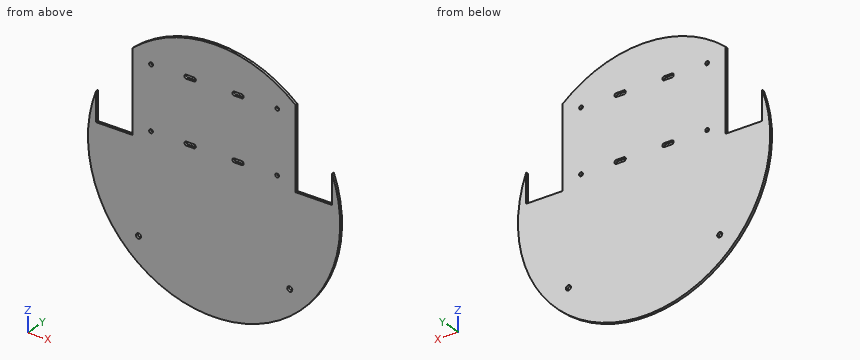
```python
from build123d import *

# Parameters (mm, degrees)
SKETCH1_R           = 1.5
SKETCH1_R_2         = 2
BOSS_EXTRUDE1_DEPTH = 2


with BuildPart() as part:
    # Sketch1 → Boss-Extrude1 (new body)
    with BuildSketch(Plane(origin=(0, 0, 0), x_dir=(1, 0, 0), z_dir=(0, 1, 0))):
        with BuildLine():
            Line((-93.5, -35.464771253), (-93.5, -12.5))
            Line((-93.5, -12.5), (-64.5, -12.5))
            Line((-64.5, -12.5), (-64.5, -76.418256981))
            ThreePointArc((-64.5, -76.418256981), (0, -100), (64.5, -76.418256981))
            Line((64.5, -76.418256981), (64.5, -12.5))
            Line((64.5, -12.5), (93.5, -12.5))
            Line((93.5, -12.5), (93.5, -35.464771253))
            ThreePointArc((93.5, -35.464771253), (0, 100), (-93.5, -35.464771253))
        make_face()
        with Locations((-50, -69)):
            Circle(SKETCH1_R, mode=Mode.SUBTRACT)
        with BuildLine():
            Line((-22, -67.5), (-16, -67.5))
            ThreePointArc((-16, -67.5), (-14.5, -69), (-16, -70.5))
            Line((-16, -70.5), (-22, -70.5))
            ThreePointArc((-22, -70.5), (-23.5, -69), (-22, -67.5))
        make_face(mode=Mode.SUBTRACT)
        with Locations((-50, -20)):
            Circle(SKETCH1_R, mode=Mode.SUBTRACT)
        with BuildLine():
            ThreePointArc((-16, -18.5), (-14.5, -20), (-16, -21.5))
            Line((-16, -21.5), (-22, -21.5))
            ThreePointArc((-22, -21.5), (-23.5, -20), (-22, -18.5))
            Line((-22, -18.5), (-16, -18.5))
        make_face(mode=Mode.SUBTRACT)
        with BuildLine():
            ThreePointArc((16, -70.5), (14.5, -69), (16, -67.5))
            Line((16, -67.5), (22, -67.5))
            ThreePointArc((22, -67.5), (23.5, -69), (22, -70.5))
            Line((22, -70.5), (16, -70.5))
        make_face(mode=Mode.SUBTRACT)
        with Locations((50, -69)):
            Circle(SKETCH1_R, mode=Mode.SUBTRACT)
        with BuildLine():
            Line((22, -21.5), (16, -21.5))
            ThreePointArc((16, -21.5), (14.5, -20), (16, -18.5))
            Line((16, -18.5), (22, -18.5))
            ThreePointArc((22, -18.5), (23.5, -20), (22, -21.5))
        make_face(mode=Mode.SUBTRACT)
        with Locations((50, -20)):
            Circle(SKETCH1_R, mode=Mode.SUBTRACT)
        with Locations((-60, 60)):
            Circle(SKETCH1_R_2, mode=Mode.SUBTRACT)
        with Locations((60, 60)):
            Circle(SKETCH1_R_2, mode=Mode.SUBTRACT)
    extrude(amount=BOSS_EXTRUDE1_DEPTH)


solid = part.part
```
Here's how the part is built. I have some questions about the finished solid (model axes, mm). Give positions to 0.01 mm unless a question says otherwise; leave off trailing zeros. Write each loop counter-clockwise with the first axis right and the second up, starting at its lowest first coordinate (ties: lowest second). Pieces come first, ordered by that corner, then holes. Notation, with made-up numbers: M -25,-28.5 L -8,-28.5 A18 cw -8,-0.5 Z; hole C 14,13.25 d11. An arc over 180 degrees is marked long. Put each result on its own line as item: value. Start each with the question number.
Item 1: Will these pins go through, and if not, where does the flat tip stop? pin 1 (2.5 mm diameter, centred on x = 50, z = 20, fed in from -Y); pin 2 (0.6 mm diameter, centred on x = 19, y = 0.5, fed in from -Z); pin 3 (0.6 mm diameter, centred on x = -20, y = 1, fed in from -Z); pin 4 (0.6 mm diameter, centred on x = 19.5, y = 1.5, fed in from -Z).
Item 2: I need wall thicknesses on L1, parallel to X at y = 1.15, z = 69; L2, parallel to X at y = 1.3, z = 33; L3, parallel to Z at x = 50, y = 0.9. Which ranges of each line are inside material? Lowest first, please. Write a range as from..to.
Item 3: If we section it at C-C, the plane x = 39.5: Write out the boundary of the cut face in (y, z), then the cut area to 3 significant figures.
Item 4: If we section it at B-B, the plane z = 65: Write out the boundary of the cut face in (x, y), then the cut area to 3 significant figures.
Item 5: If we section it at A-A, the plane y = 0.35: Count the separate pieces of the cut face and the enclosed holes in it, then the cut area to 3 significant figures.
Values:
1. pin 1: through
1. pin 2: z = -98.24
1. pin 3: z = -98.04
1. pin 4: z = -98.14
2. L1: -64.5..-51.5, -48.5..-23.5, -14.5..14.5, 23.5..48.5, 51.5..64.5
2. L2: -94.4..-93.5, -64.5..64.5, 93.5..94.4
2. L3: -86.6..18.5, 21.5..67.5, 70.5..86.6
3. outline: M 0,-91.87 L 2,-91.87 L 2,91.87 L 0,91.87 Z
3. area: 367 mm²
4. outline: M -64.5,0 L 64.5,0 L 64.5,2 L -64.5,2 Z
4. area: 258 mm²
5. separate pieces: 1
5. enclosed holes: 10
5. area: 28,500 mm²
